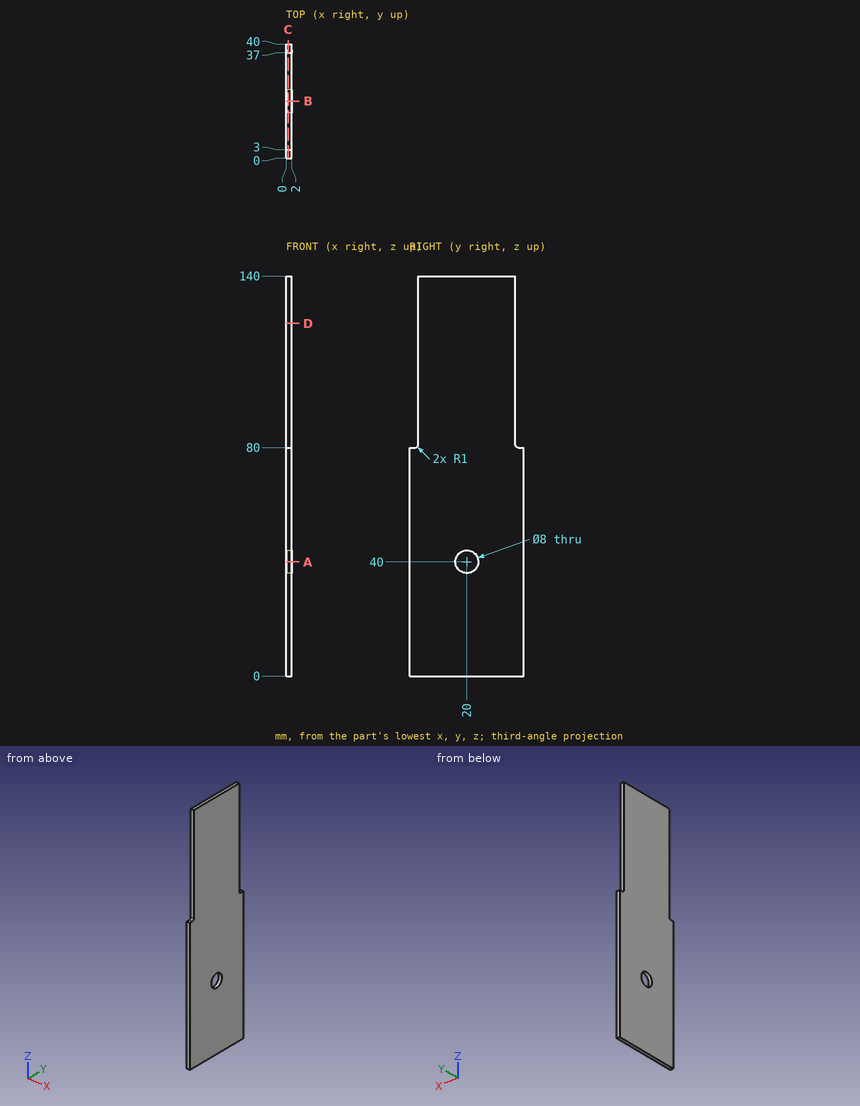
Answer from the drawing. Dimensions are ordinates in mm from the lowest x, y and z of the part. Give positions to 0.01 mm unless a question says otherwise; leave off trailing zeros. Write each loop counter-clockwise with the first axis right and the second up, starting at its lowest first coordinate (ties: lowest second). Pieces come first, ordered by that corner, then holes.
1) Given P1, Ø7, axis at y = 20, z = 40, coming from the +X side; P2, Ø0.6, axis at x = 1, y = 38.5, coming from the +Z side, each flat-ended and moving along its own axis, determine where each tip first touches the part or whether it passes through.
2) Section C-C (x = 0.7) is taken. Write down the section's boundary in (y, z), and give its area (3 significant figures).
3) Find the intervals of material crossed by L1, parallel to Y at x = 0.9, z = 40; L2, parallel to Y at x = 0.4, z = 104; L3, parallel to Z at x = 0.35, y = 23.5, in increasing order.
4) Section A-A (z = 40) is taken. Write down the section's boundary in (x, y), and give its area (3 significant figures).
5) Section B-B (y = 20) is taken. Write down the section's boundary in (x, z).
6) Section D-D (z = 123.5) is taken. Write down the section's boundary in (x, y).
Response:
1. P1: passes through
1. P2: stops at z = 80
2. outline: (0, 0) - (40, 0) - (40, 80) - (38, 80) arc R1 cw to (37, 81) - (37, 140) - (3, 140) - (3, 81) arc R1 cw to (2, 80) - (0, 80) - close; hole circle Ø8 at (20, 40)
2. area: 5,190 mm2
3. L1: y = 0 to 16, 24 to 40
3. L2: y = 3 to 37
3. L3: z = 0 to 38.06, 41.94 to 140
4. outline: (0, 0) - (2, 0) - (2, 16) - (0, 16) - close; (0, 24) - (2, 24) - (2, 40) - (0, 40) - close
4. area: 64.0 mm2
5. outline: (0, 0) - (2, 0) - (2, 36) - (0, 36) - close; (0, 44) - (2, 44) - (2, 140) - (0, 140) - close
6. outline: (0, 3) - (2, 3) - (2, 37) - (0, 37) - close
